Geometry check sheet. Reference: the model listing, model coordinates, mm. Face numbers are marked on the shaded views. A direction names the side the tool comes from. Round coordinates to 2 decimals unless told otherwise and drop trailing zeros. Write each loop counter-clockwise with the first axis right and the second up, starting at its lowest first coordinate (ties: lowest second). Pieces come first, ordered by that corner, then holes.
from build123d import *

# Parameters (mm, degrees)
BOSS_EXTRUDE1_DEPTH = 7


with BuildPart() as part:
    # Sketch1 → Boss-Extrude1 (new body)
    with BuildSketch(Plane.XY):
        with BuildLine():
            Line((-13.5, -1.520113715), (-13.5, -0.377223398))
            ThreePointArc((-13.5, -0.377223398), (-12.914213562, 1.036990164), (-11.5, 1.622776602))
            Line((-11.5, 1.622776602), (11.5, 1.622776602))
            ThreePointArc((11.5, 1.622776602), (12.914213562, 1.036990164), (13.5, -0.377223398))
            Line((13.5, -0.377223398), (13.5, -1.520113715))
            ThreePointArc((13.5, -1.520113715), (13.034625892, -4.535227161), (11.681818182, -7.269709461))
            ThreePointArc((11.681818182, -7.269709461), (5.594183484, -19.574879811), (3.5, -33.142890317))
            Line((3.5, -33.142890317), (3.5, -40.642890317))
            Line((3.5, -40.642890317), (-3.5, -40.642890317))
            Line((-3.5, -40.642890317), (-3.5, -33.142890317))
            ThreePointArc((-3.5, -33.142890317), (-5.594183484, -19.574879811), (-11.681818182, -7.269709461))
            ThreePointArc((-11.681818182, -7.269709461), (-13.034625892, -4.535227161), (-13.5, -1.520113715))
        make_face()
    boss_extrude1 = extrude(amount=BOSS_EXTRUDE1_DEPTH)

    # Mirror1: Boss-Extrude1 across plane
    add(boss_extrude1.mirror(Plane(origin=(3.5, -40.642890317, 7), x_dir=(0, 0, 1), z_dir=(0, 1, 0))))


solid = part.part
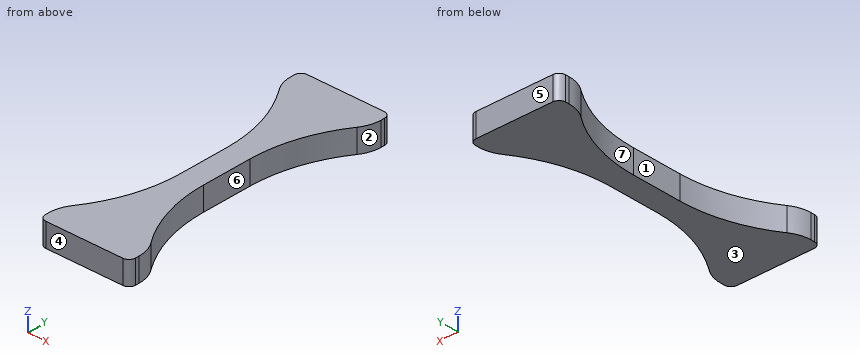
1. Access from +Z, -Z, +X, -X, +Y, -Y to the whole of each face (thin tool, end or side, straight path). Record for the marked faces 5, 6 and 7.
2. Release check for a two-part mould opening along Y. For the marked faces 1, 2, 3 and 4 record: +Y half, -Y half, draft (parallel to the pull), parting line (faces both ways), or undercut.
3. Section check D-D (x = -4.5). Record the cut outline in (y, z), plus the area to 3 significant figures.
4. Section check C-C (y = -18). Record the cut outline in (x, z).
5. Scan lines: line 1 along X through (y, z) = (-35.5, 6.75); line 2 along Y through (x, z) = (-9.5, 5); line 3 along Y through (x, z) = (-8, 4.25). Record each from-to range of solid material in increasing order.
6. Section check B-B (x = 7.5). Record the cut outline in (y, z), plus the area to 3 significant figures.
7. Depth check by flat-ended pin: pin 1 Ø1 at (y, z) = (-33.5, 4.5) entering from -X; pin 2 Ø2 at (y, z) = (-44, 4) entering from +X; pin 3 Ø4 at (y, z) = (-29, 5.5) entering from -X. Enter the tip coordinate at first touch or a pass-through.
8. Section check A-A (z = 2.5). Record the cut outline in (x, y).
Results below:
1. face 5: +Z, -Z, +X, -X, +Y
1. face 6: +Z, -Z, +X
1. face 7: +Z, -Z, -X
2. face 1: undercut
2. face 2: undercut
2. face 3: draft
2. face 4: -Y half
3. outline: (-82.91, 0) - (-57.58, 0) - (-57.58, 7) - (-82.91, 7) - close; (-23.71, 0) - (1.62, 0) - (1.62, 7) - (-23.71, 7) - close
3. area: 355 mm2
4. outline: (-6.12, 0) - (6.12, 0) - (6.12, 7) - (-6.12, 7) - close
5. line 1: x = -3.5 to 3.5
5. line 2: y = -82.91 to -70.59, -10.69 to 1.62
5. line 3: y = -82.91 to -67.76, -13.53 to 1.62
6. outline: (-82.91, 0) - (-66.69, 0) - (-66.69, 7) - (-82.91, 7) - close; (-14.6, 0) - (1.62, 0) - (1.62, 7) - (-14.6, 7) - close
6. area: 227 mm2
7. pin 1: stops at x = -3.5
7. pin 2: stops at x = 3.5
7. pin 3: stops at x = -3.92
8. outline: (-13.5, -80.91) arc R2 ccw to (-11.5, -82.91) - (11.5, -82.91) arc R2 ccw to (13.5, -80.91) - (13.5, -79.77) arc R10 ccw to (11.68, -74.02) arc R45 cw to (3.5, -48.14) - (3.5, -33.14) arc R45 cw to (11.68, -7.27) arc R10 ccw to (13.5, -1.52) - (13.5, -0.38) arc R2 ccw to (11.5, 1.62) - (-11.5, 1.62) arc R2 ccw to (-13.5, -0.38) - (-13.5, -1.52) arc R10 ccw to (-11.68, -7.27) arc R45 cw to (-3.5, -33.14) - (-3.5, -48.14) arc R45 cw to (-11.68, -74.02) arc R10 ccw to (-13.5, -79.77) - close
